Autodesk Inventor part; units mm, degrees
ref_plane "YZ Plane" through (0, 0, 0) normal (1, 0, 0) x (0, 1, 0)
ref_plane "XZ Plane" through (0, 0, 0) normal (0, 1, 0) x (-1, 0, 0)
ref_plane "XY Plane" through (0, 0, 0) normal (0, 0, 1) x (1, 0, 0)
sketch "Szkic1" plane through (0, 0, 0) normal (0, 0, 1) x (1, 0, 0)
  line L0 (-20, 16) -> (20, 16)
  line L1 (25, 11) -> (25, -11)
  line L2 (20, -16) -> (-20, -16)
  line L3 (-25, -11) -> (-25, 11)
  line L4 (-25, 16) -> (25, -16) construction
  line L5 (25, 16) -> (-25, -16) construction
  arc A0 (25, 11) -> (20, 16) centre (20, 11) ccw
  arc A1 (20, -16) -> (25, -11) centre (20, -11) ccw
  arc A2 (-25, -11) -> (-20, -16) centre (-20, -11) ccw
  arc A3 (-20, 16) -> (-25, 11) centre (-20, 11) ccw
  circle A4 centre (-20, 11) radius 3
  circle A5 centre (-20, -11) radius 3
  point P0 (0, 0)
  dimension "d0" = 50
  dimension "d1" = 32
  dimension "d3" = 5
  dimension "d4" = 5
  dimension "d5" = 6
  dimension "d6" = 6
extrude "Wyciągnięcie proste1" add sketch "Szkic1" along normal blind 10
sketch "Szkic2" plane through (0, 0, 10) normal (0, 0, 1) x (1, 0, 0)
  line L0 (-4, -12) -> (4, -12)
  line L1 (4, -12) -> (4, 12)
  line L2 (4, 12) -> (-4, 12)
  line L3 (-4, 12) -> (-4, -12)
  line L4 (-4, -12) -> (4, 12) construction
  line L5 (4, -12) -> (-4, 12) construction
  point P0 (0, 0)
  dimension "d9" = 8
  dimension "d10" = 24
extrude "Wyciągnięcie proste2" add sketch "Szkic2" along normal blind 18
sketch "Szkic3" plane through (4, -12, 10) normal (1, 0, 0) x (0, 0, -1)
  line L0 (0, 24) -> (-18, 24) construction
  line L1 (-9, 24) -> (-9, 0) construction
  line L2 (0, 0) -> (-18, 0) construction
  line L3 (-18, 0) -> (-18, 24) construction
  line L4 (-18, 12) -> (0, 12) construction
  line L5 (0, 23) -> (0, 1) construction
  circle A0 centre (-10, 12) radius 5
  line L6 (-18, 12) -> (-10, 12) construction
  point P0 (10, 12)
  dimension "d13" = 10
  dimension "d28" = 8
extrude "Wyciągnięcie proste3" cut sketch "Szkic3" against normal up to next
fillet "Zaokrąglenie1" radius 2 4 edges at (0, 12, 10) (4, 0, 10) (0, -12, 10) (-4, 0, 10)
fillet "Zaokrąglenie2" radius 5 2 edges at (0, -12, 28) (0, 12, 28)
sketch "Szkic4" plane through (-20, -16, 0) normal (0, -1, 0) x (1, 0, 0)
  line L0 (40, 0) -> (40, 10) construction
  line L1 (45, 0) -> (40, 0)
  line L2 (45, 0) -> (35, 0)
  line L3 (35, 0) -> (30, 0)
  line L4 (30, 0) -> (30, 3)
  line L5 (30, 3) -> (35, 3)
  line L6 (35, 3) -> (35, 0)
  dimension "d23" = 10
  dimension "d24" = 5
  dimension "d25" = 3
extrude "Wyciągnięcie proste4" cut sketch "Szkic4" against normal up to next
properties part number "Bartosz_Zukowski_IP_model_4.ipj"
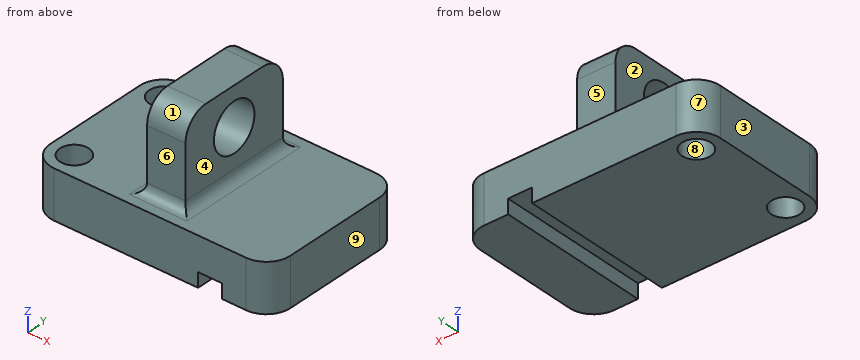
Source: CAD feature listing. Evaluate the final solid. Frame: model axes, mm. Face numbers are marked on the shaded views. A direction names the side the tool comes from. Give positions to 0.01 mm unless a question says otherwise; leave off trailing zeros. Loops run counter-clockwise (first coordinate to the right, second up) from the corner with the lowest first, then second, coordinate; pieces in that order, holes last. Notation, with made-up numbers: (20, -30) -> (68, -30) arc R26 cw to (68, 5) -> close; hole circle Ø10 at (37, -37). An arc over 180 degrees is marked (long way). Use a Markdown table: item, result. Add a question column.
(1) Ray query, line 1 (Y direction, x = -20, z = 6.5); line 2 (Y direction, x = -3.5, z = 20); line 3 (X direction, y = 5, z = 20.75). Return the intervals inside material, ascending.
(2) Section query B-B (y = -1). Output: boundary loops of the cut face in (x, z).
(3) Section query A-A (z = 20). Output: boundary loops of the cut face in (x, y).
(4) Section query D-D (x = -19). Output: boundary loops of the cut face in (y, z).
(5) Section query C-C (z = 7.5). Output: boundary loops of the cut face in (x, y).
(6) Pull-direction query (X, two-part tool) for the marked faces 6, 7, 8 and 9; classes: +X half, -X half, draft (parallel to the pull), parting line (faces both ways), or undercut.
(7) First-contact query: pin 1 Ø4 at (x, z) = (0.5, 18.5) entering from +Y; pin 2 Ø7 at (x, y) = (-20, 11) entering from -Z; pin 3 Ø5 at (y, z) = (-1.5, 16.5) entering from +X; pin 4 Ø6 at (x, y) = (-19.5, 9.5) entering from +Z. Flat tips, straight axial feed; report the tip coordinate or a pass-through.
(8) Access query for the marked faces 1, 2, 3, 4 and 5. Directions: +Z, -Z, +X, -X, +Y, -Y. A direction counts if a zero-diameter tool reaches every point of the face in a straight line with its end or side. Return the directions, or none.
Checked values:
| question | item | result |
|---|---|---|
| 1 | line 1 | -16 to -14, -8 to 8, 14 to 16 |
| 1 | line 2 | -12 to -5, 5 to 12 |
| 1 | line 3 | -4 to 4 |
| 2 | outline | (-25, 0) -> (10, 0) -> (10, 3) -> (15, 3) -> (15, 0) -> (25, 0) -> (25, 10) -> (6, 10) arc R2 cw to (4, 12) -> (4, 15.1) -> (-4, 15.1) -> (-4, 12) arc R2 cw to (-6, 10) -> (-25, 10) -> close; (-4, 24.9) -> (4, 24.9) -> (4, 28) -> (-4, 28) -> close |
| 3 | outline | (-4, -12) -> (4, -12) -> (4, -5) -> (-4, -5) -> close; (-4, 5) -> (4, 5) -> (4, 12) -> (-4, 12) -> close |
| 4 | outline | (-16, 0) -> (-13.83, 0) -> (-13.83, 10) -> (-16, 10) -> close; (-8.17, 0) -> (8.17, 0) -> (8.17, 10) -> (-8.17, 10) -> close; (13.83, 0) -> (16, 0) -> (16, 10) -> (13.83, 10) -> close |
| 5 | outline | (-25, -11) arc R5 ccw to (-20, -16) -> (20, -16) arc R5 ccw to (25, -11) -> (25, 11) arc R5 ccw to (20, 16) -> (-20, 16) arc R5 ccw to (-25, 11) -> close; hole circle Ø6 at (-20, -11); hole circle Ø6 at (-20, 11) |
| 6 | face 6 | draft |
| 6 | face 7 | -X half |
| 6 | face 8 | undercut |
| 6 | face 9 | +X half |
| 7 | pin 1 | y = 12 |
| 7 | pin 2 | z = 0 |
| 7 | pin 3 | x = 4 |
| 7 | pin 4 | z = 10 |
| 8 | face 1 | +Z, +X, -X, -Y |
| 8 | face 2 | +Z, -X, +Y, -Y |
| 8 | face 3 | +Z, -Z, -X, +Y, -Y |
| 8 | face 4 | +Z, +X, +Y, -Y |
| 8 | face 5 | +Z, +X, -X, +Y |
